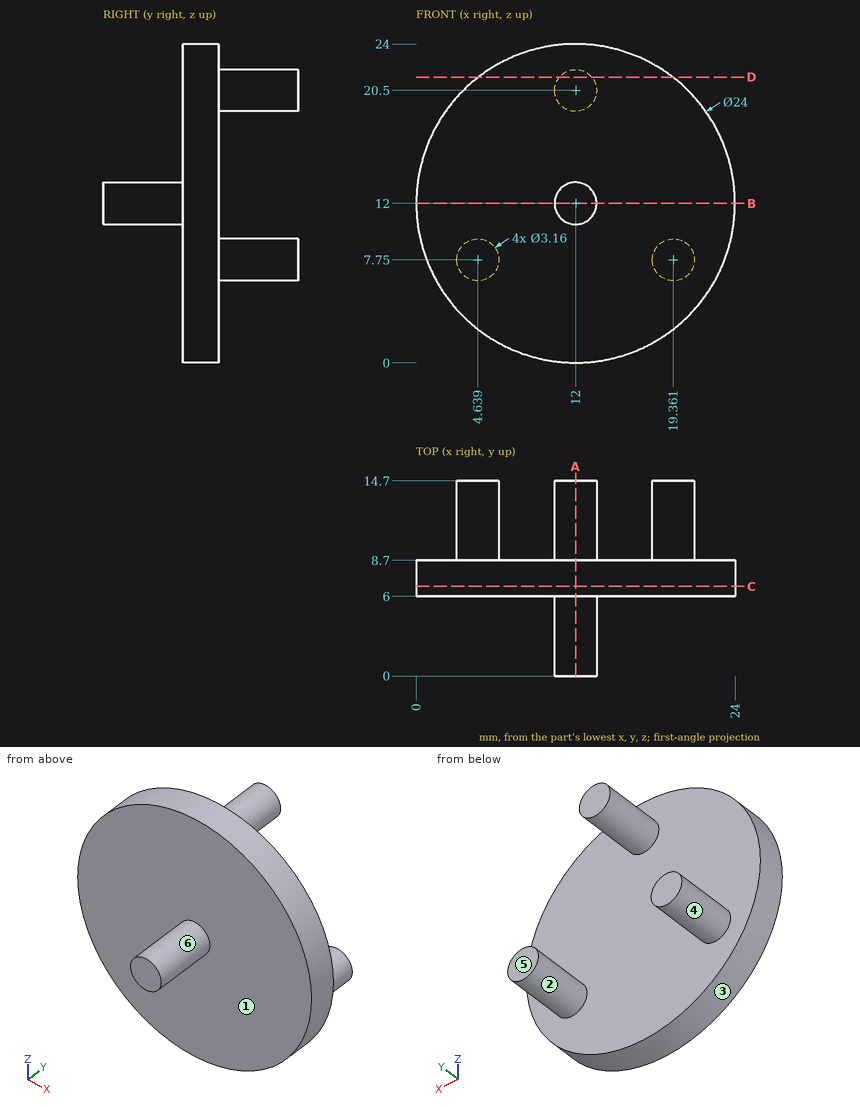
The figure shows three views and two pictorial views of one solid part (mm, origin at its lowest corner). Answer the questions. A direction names the side the tool comes from. Coordinates: 2 decimals unless noted, no trailing zeros. Loops run counter-clockwise (first coordinate to the right, second up) from the corner with the lowest first, then second, coordinate; pieces in that order, holes last. Notation, with made-up numbers: (56.5, 64) -> (90.5, 64) arc R30 cw to (90.5, 103) -> close; hole circle Ø9 at (52, 45.5). An arc over 180 degrees is marked (long way). Use one line per item in the form item = value. Start each with the question number.
Item 1: The part is cut by section B-B on z = 12. Determine the outline of the cut face in (x, y).
Item 2: The part is cut by section D-D on z = 21.5. Determine the outline of the cut face in (x, y).
Item 3: Flat-ended cylindrical pins translate along their axes: pin 1 Ø4 at (y, z) = (7, 15) entering from +X; pin 2 Ø8 at (x, z) = (17, 16.5) entering from +Y; pin 3 Ø8 at (y, z) = (3.5, 4) entering from -X. Find the tip coordinate at first contact, or state that the pin passes through.
Item 4: A tool of negligible diameter and unlimited length cuts with its end or side. For the marked faces 4, 5 and 6, from which of +Z, -Z, +X, -X, +Y, -Y can it reach the whole face along a straight path? Write none if from no direction.
Item 5: The part is cut by section A-A on x = 12. Determine the outline of the cut face in (y, z), then the cut area to 3 significant figures.
Item 6: The part is cut by section C-C on y = 6.75. Determine the outline of the cut face in (x, z).
Item 7: Consider L1, parallel to Y at x = 4, z = 12.75; L2, parallel to Y at x = 12.75, z = 11.75; L3, parallel to X at y = 7.75, z = 20 (1 decimal). Determine where each line is inside the solid, lowest interval first. Write a range as [from, to].
Item 8: The mould has two halves that part along X. Classify the marked faces 1, 2 and 3: released by +X, released by -X, zero draft, split by the parting line, or undercut.
Answer key:
q1.outline = (0, 6) -> (10.42, 6) -> (10.42, 0) -> (13.58, 0) -> (13.58, 6) -> (24, 6) -> (24, 8.7) -> (0, 8.7) -> close
q2.outline = (4.67, 6) -> (19.33, 6) -> (19.33, 8.7) -> (13.22, 8.7) -> (13.22, 14.7) -> (10.78, 14.7) -> (10.78, 8.7) -> (4.67, 8.7) -> close
q3.pin_1 = 23.96
q3.pin_2 = 8.7
q3.pin_3 = 1.04
q4.face_4 = +Y
q4.face_5 = +Z, -Z, +X, -X, +Y
q4.face_6 = -Y
q5.outline = (0, 10.42) -> (6, 10.42) -> (6, 0) -> (8.7, 0) -> (8.7, 18.92) -> (14.7, 18.92) -> (14.7, 22.08) -> (8.7, 22.08) -> (8.7, 24) -> (6, 24) -> (6, 13.58) -> (0, 13.58) -> close
q5.area = 103 mm2
q6.outline = circle Ø24 at (12, 12)
q7.L1 = [6, 8.7]
q7.L2 = [0, 8.7]
q7.L3 = [3.1, 20.9]
q8.face_1 = zero draft
q8.face_2 = undercut
q8.face_3 = split by the parting line
